For this review, take the finished solid that the model builds, in its own axes (mm). A direction names the side the tool comes from. Coordinates: 2 decimals unless noted, no trailing zeros. Loops run counter-clockwise (first coordinate to the right, second up) from the corner with the lowest first, then second, coordinate; pieces in that order, holes last.
```python
from build123d import *

# Parameters (mm, degrees)
CUT_EXTRUDE1_DEPTH  = 4
SKETCH3_R           = 12.483239851
BOSS_EXTRUDE1_DEPTH = 63
CUT_EXTRUDE2_DEPTH  = 4
CHAMFER1_SIZE       = 1


with BuildPart() as part:
    # Sketch1 → Revolve1 (revolve)
    with BuildSketch(Plane.XY, mode=Mode.PRIVATE) as revolve1_sk:
        Polygon((-63.043142844, 0), (-63.043142844, 12.483239851), (-20.551205143, 12.483239851), (-20.544749915, 16.500001291), (-19.543142844, 17.5), (14.456857156, 17.5), (14.456857156, 21.5), (15.456857156, 22.5), (18.956857156, 22.5), (19.956857156, 21.5), (19.956857156, 17.5), (34.956857156, 17.5), (36.956857156, 15.5), (36.956857156, 0), align=None)
    revolve(revolve1_sk.sketch.rotate(Axis((-79.289099526, 0, 0), (1, 0, 0)), 90), axis=Axis((-79.289099526, 0, 0), (1, 0, 0)))

    # Sketch2 → Cut-Extrude1 (cut)
    with BuildSketch(Plane(origin=(0, 17.5, 0), x_dir=(1, 0, 0), z_dir=(0, 1, 0))):
        with BuildLine():
            Line((-15.033175355, 4), (9.966824645, 4))
            ThreePointArc((9.966824645, 4), (13.966824645, 0), (9.966824645, -4))
            Line((9.966824645, -4), (-15.033175355, -4))
            ThreePointArc((-15.033175355, -4), (-19.033175355, 0), (-15.033175355, 4))
        make_face()
    extrude(amount=-CUT_EXTRUDE1_DEPTH, mode=Mode.SUBTRACT)

    # Sketch3 → Boss-Extrude1 (add)
    with BuildSketch(Plane.ZY.offset(63.043142844)):
        Circle(SKETCH3_R)
    extrude(amount=BOSS_EXTRUDE1_DEPTH)

    # Sketch4 → Cut-Extrude2 (cut)
    with BuildSketch(Plane(origin=(0, 12.483239851, 0), x_dir=(1, 0, 0), z_dir=(0, 1, 0))):
        with BuildLine():
            Line((-107.043142844, 4), (-82.043142844, 4))
            ThreePointArc((-82.043142844, 4), (-78.043142844, 0), (-82.043142844, -4))
            Line((-82.043142844, -4), (-107.043142844, -4))
            ThreePointArc((-107.043142844, -4), (-111.043142844, 0), (-107.043142844, 4))
        make_face()
    extrude(amount=-CUT_EXTRUDE2_DEPTH, mode=Mode.SUBTRACT)

    # Chamfer1
    chamfer1_edges = [part.edges().sort_by_distance(p)[0] for p in [
        (-126.043142844, 0, -12.483239851),
    ]]
    chamfer(chamfer1_edges, length=CHAMFER1_SIZE)


solid = part.part
```
Q1. Consider section C-C (x = -68.5). State the section outline as (y, z) points.
Q2. Machinability: for faces 1 (the face through (27.562, 17.084, -3.794)), 2 (the face through (-2.305, -14.756, 9.408)), 3 (the face through (17.231, 19.961, 10.382)), 4 (the face through (-2, 15, 4)), which of the approach directions +Z, -Z, +X, -X, +Y, -Y give a long, thin tool a straight path to every point of the face, cutting with its end or side? Answer none if there is none.
Q3. Wall thickness on probe 1 along X at (y, z) = (14.5, -15); probe 2 along Z at (x, y) = (-10, 15.5); probe 3 along Z at (x, y) = (-56, 11): over which ranges is each line inside the solid? List them lowest first.
Q4. The part is to be moulded in two halves that separate along Z. For faces 5 (the face through (-72.066, -12.186, -2.706)), 6 (the face through (-126.043, 0, 0)), 7 (the face through (-3, 15, -4)), 8 (the face through (-2, 13.5, 0)), say which applies: +Z half, -Z half, draft (parallel to the pull), parting line (faces both ways), or undercut.
Q5. Consider section B-B (y = 0). State the section outline as (x, z) points.
Q6. For pin 1 Ø4 at (x, z) = (1, 10) entering from -Y; pin 2 Ø1 at (x, z) = (-70, -5) entering from +Y; pin 3 Ø1.8 at (x, y) = (-6.5, 16) entering from -Z, all flat-tipped, find the tip position at first contact; note any pin that passes through.
Model answer:
1. outline: circle Ø24.97 at (0, 0)
2. face 1: +X
2. face 2: -X
2. face 3: +X, -X
2. face 4: +Y
3. probe 1: x = 14.46 to 19.96
3. probe 2: z = -8.12 to -4, 4 to 8.12
3. probe 3: z = -5.9 to 5.9
4. face 5: parting line
4. face 6: draft
4. face 7: undercut
4. face 8: undercut
5. outline: (-126.04, -11.48) - (-125.04, -12.48) - (-20.55, -12.48) - (-20.54, -16.5) - (-19.54, -17.5) - (14.46, -17.5) - (14.46, -21.5) - (15.46, -22.5) - (18.96, -22.5) - (19.96, -21.5) - (19.96, -17.5) - (34.96, -17.5) - (36.96, -15.5) - (36.96, 15.5) - (34.96, 17.5) - (19.96, 17.5) - (19.96, 21.5) - (18.96, 22.5) - (15.46, 22.5) - (14.46, 21.5) - (14.46, 17.5) - (-19.54, 17.5) - (-20.54, 16.5) - (-20.55, 12.48) - (-125.04, 12.48) - (-126.04, 11.48) - close
6. pin 1: stops at y = -15.56
6. pin 2: stops at y = 11.64
6. pin 3: stops at z = -8.85
